For this review, take the finished solid that the model builds, in its own axes (mm). Face numbers are marked on the shaded views. A direction names the side the tool comes from. Coordinates: 2 decimals unless noted, no trailing zeros. Loops run counter-clockwise (first coordinate to the right, second up) from the corner with the lowest first, then second, coordinate; pieces in that order, holes last. Notation, with made-up numbers: (-13, 55.5) -> (38, 55.5) arc R21 ccw to (38, 85.5) -> close; hole circle Ø6 at (-5, 1.25). An arc over 180 degrees is marked (long way). Use a Markdown table: item, result.
from build123d import *

# Parameters (mm, degrees)
F1_DEPTH       = 18
F4_D           = 4.4
F4_CBORE_D     = 8.25
F4_CBORE_DEPTH = 4
F5_R           = 8.99999
F6_R           = 2
F7_D           = 3.3
F7_CBORE_D     = 6.5
F7_CBORE_DEPTH = 3
F9_DEPTH       = 3


# Not quite as in the source:
# - a fillet or chamfer is up to 0.001 mm smaller than in the source, because OpenCascade refuses the exact size


with BuildPart() as f1:
    # F0 (on Right) → F1 (new body)
    with BuildSketch(Plane.YZ):
        with BuildLine():
            Line((0, 6), (0, 0))
            Line((0, 0), (48, 0))
            Line((48, 0), (48, 6))
            Line((48, 6), (34, 6))
            ThreePointArc((34, 6), (32.5857864376, 6.5857864376), (32, 8))
            Line((32, 8), (32, 24))
            Line((32, 24), (24.75, 24))
            Line((24.75, 24), (24.75, 12.9434299833))
            ThreePointArc((24.75, 12.9434299833), (24, 3), (23.25, 12.9434299833))
            Line((23.25, 12.9434299833), (23.25, 24))
            Line((23.25, 24), (16, 24))
            Line((16, 24), (16, 8))
            ThreePointArc((16, 8), (15.4142135624, 6.5857864376), (14, 6))
            Line((14, 6), (0, 6))
        make_face()
    extrude(amount=F1_DEPTH)

    # F4 (through all)
    with Locations(Plane.XY.offset(6)):
        with Locations((9, 9), (9, 39)):
            CounterBoreHole(F4_D / 2, F4_CBORE_D / 2, F4_CBORE_DEPTH)

    # F5 (radius 9 in the source; OpenCascade refuses exactly that, so slightly less here)
    f5_edges = [f1.edges().sort_by_distance(p)[0] for p in [
        (18, 0, 3),
        (0, 0, 3),
        (18, 48, 3),
        (0, 48, 3),
        (0, 28.375, 24),
        (0, 19.625, 24),
        (18, 19.625, 24),
        (18, 28.375, 24),
    ]]
    fillet(f5_edges, radius=F5_R)

    # F6
    f6_edges = [f1.edges().sort_by_distance(p)[0] for p in [
        (18, 11.499995, 6),
        (18, 36.500005, 6),
    ]]
    fillet(f6_edges, radius=F6_R)

    # F7 (through all)
    with Locations(Plane.XZ.offset(-16)):
        with Locations((9, 15)):
            CounterBoreHole(F7_D / 2, F7_CBORE_D / 2, F7_CBORE_DEPTH)

    # F8 (on face) → F9 (cut)
    with BuildSketch(Plane(origin=(0, 32, 0), x_dir=(-1, 0, 0), z_dir=(0, 1, 0))):
        Polygon((-6, 13.2679491924), (-6, 16.7320508076), (-9, 18.4641016151), (-12, 16.7320508076), (-12, 13.2679491924), (-9, 11.5358983849), align=None)
    extrude(amount=-F9_DEPTH, mode=Mode.SUBTRACT)


solid = f1.part
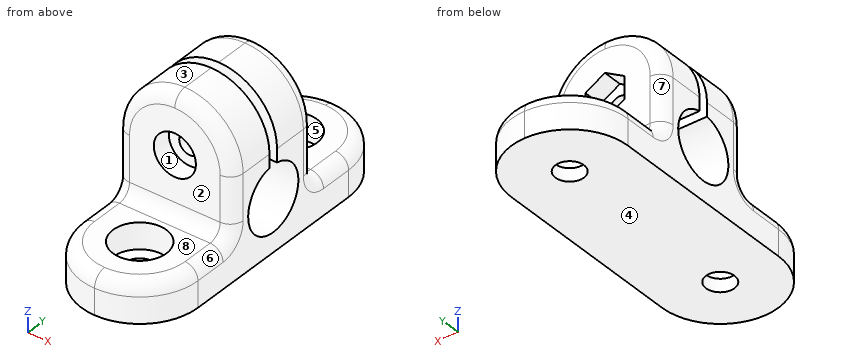
(1) For pin 1 Ø5 at (x, z) = (9, 15) entering from +Y; pin 2 Ø4.5 at (x, z) = (9, 15) entering from -Y; pin 3 Ø3 at (x, z) = (10.5, 10) entering from -Y, all flat-tipped, find the tip position at first contact; note any pin that passes through.
Found:
| item | result |
|---|---|
| pin 1 | stops at y = 29 |
| pin 2 | stops at y = 19 |
| pin 3 | stops at y = 16 |
(2) For line 1 along Y through (x, z) = (9, 1.05); line 2 along Y through (x, z) = (11.25, 13.5); line 3 along Z through (x, y) = (9, 17.8), list the stretches that pass through material, from the lowest coordinate up.
Found:
| item | result |
|---|---|
| line 1 | y = 0 to 6.8, 11.2 to 36.8, 41.2 to 48 |
| line 2 | y = 19 to 23.25, 24.75 to 29 |
| line 3 | z = 0 to 11.75, 18.25 to 23.99 |
(3) Mouldability with a two-part tool opening along Z and no side actions: class the marked faces 1, 2, 3 and 4 as pulls with the +Z half, pulls with the -Z half, needs draft (parallel to the pull), parting line crosses it, or undercut.
Found:
| item | result |
|---|---|
| face 1 | undercut |
| face 2 | needs draft |
| face 3 | pulls with the +Z half |
| face 4 | pulls with the -Z half |
(4) Take a section at B-B on y = 21.5. State how many separate pieces and enclosed holes the cut face has, plus the area to 3 significant figures.
Found:
| item | result |
|---|---|
| separate pieces | 2 |
| enclosed holes | 1 |
| area | 233 mm^2 |
(5) For the marked faces 5, 6, 7 and 8, list the 3-axis set-ups (+Z, -Z, +X, -X, +Y, -Y) from which the entire face can be reached by the end or side of a thin tool; tool diameter is ignored.
Found:
| item | result |
|---|---|
| face 5 | +Z |
| face 6 | +Z, +X, -Y |
| face 7 | +Z, -X, +Y |
| face 8 | +Z, +X, -X, -Y |
(6) Take a section at A-A on y = 10.5. Write out the cut boundary in (x, z), plus the area to 3 significant figures.
Found:
| item | result |
|---|---|
| outline | (0, 0) -> (7.39, 0) -> (7.39, 2) -> (5.16, 2) -> (5.16, 6) -> (2, 6) arc R2 ccw to (0, 4) -> close; (10.61, 0) -> (18, 0) -> (18, 4) arc R2 ccw to (16, 6) -> (12.84, 6) -> (12.84, 2) -> (10.61, 2) -> close |
| area | 69.1 mm^2 |
